Build history of the part. All positions in model axes, mm. A direction names the side the tool comes from. Round coordinates to 2 decimals unless told otherwise and drop trailing zeros. Write each loop counter-clockwise with the first axis right and the second up, starting at its lowest first coordinate (ties: lowest second). Pieces come first, ordered by that corner, then holes. Notation, with made-up numbers: (-20, 10.25) -> (2, 10.25) arc R19 cw to (2, 33.25) -> close; hole circle Ø1 at (53, -35). An arc over 180 degrees is marked (long way). Answer in a Markdown table with one row per item.
```python
from build123d import *

# Parameters (mm, degrees)
SKETCH1_R             = 3.81
BOSS_EXTRUDE1_DEPTH   = 127
F_2_64_TAPPED_HOLE1_D = 1.778
F_2_64_TAPPED_HOLE2_D = 1.778
LPATTERN1_COUNT       = 2
LPATTERN1_PITCH       = 25.4
LPATTERN2_COUNT       = 2
LPATTERN2_PITCH       = 25.4
SKETCH22_R            = 3.81
SKETCH22_R_2          = 2.38125
CUT_EXTRUDE1_DEPTH    = 12.7


with BuildPart() as part:
    # Sketch1 → Boss-Extrude1 (new body)
    with BuildSketch(Plane(origin=(0, 0, 0), x_dir=(1, 0, 0), z_dir=(0, 1, 0))):
        with Locations(Location((0, 0, 0), (0, 0, 270))):
            Circle(SKETCH1_R)
    extrude(amount=BOSS_EXTRUDE1_DEPTH)

    # #2-64 Tapped Hole1 (through all)
    with Locations(Plane(origin=(3.81, 0, 0), x_dir=(0, 0, -1), z_dir=(1, 0, 0))):
        with Locations((0, 76.2)):
            f_2_64_tapped_hole1 = Hole(F_2_64_TAPPED_HOLE1_D / 2)

    # #2-64 Tapped Hole2 (through all)
    with Locations(Plane(origin=(0, 0, 3.81), x_dir=(0, -1, 0), z_dir=(0, 0, 1))):
        with Locations((-88.9, 0)):
            f_2_64_tapped_hole2 = Hole(F_2_64_TAPPED_HOLE2_D / 2)

    # LPattern1: #2-64 Tapped Hole1 ×2
    with Locations(*[(0, i * LPATTERN1_PITCH, 0) for i in range(1, LPATTERN1_COUNT)]):
        add(f_2_64_tapped_hole1, mode=Mode.SUBTRACT)

    # LPattern2: #2-64 Tapped Hole2 ×2
    with Locations(*[(0, i * LPATTERN2_PITCH, 0) for i in range(1, LPATTERN2_COUNT)]):
        add(f_2_64_tapped_hole2, mode=Mode.SUBTRACT)

    # Sketch22 → Cut-Extrude1 (cut)
    with BuildSketch(Plane.XZ):
        with Locations(Location((0, 0, 0), (0, 0, 270))):
            Circle(SKETCH22_R)
        with Locations(Location((0, 0, 0), (0, 0, 270))):
            Circle(SKETCH22_R_2, mode=Mode.SUBTRACT)
    extrude(amount=-CUT_EXTRUDE1_DEPTH, mode=Mode.SUBTRACT)


solid = part.part
```
Q1. Which spindle directions (+Z, -Z, +X, -X, +Y, -Y) get a long thin tool onto all of the face, cutting with end or side? Do faces 1 (the flat face through (0, 0, 0)), 2 (the flat face through (-2, 12.7, 2)). Say none if no direction does.
A:
| item | result |
|---|---|
| face 1 | +Z, -Z, +X, -X, -Y |
| face 2 | -Y |
Q2. Drop flat-ended pins along their axis: P1, Ø2, axis at x = 0, y = 114.3, coming from the -Z side; P2, Ø2, axis at x = 2.5, y = 35, coming from the -Z side; P3, Ø2, axis at y = 83.5, z = 2, coming from the +X side. Give the stop position or say it passes through.
A:
| item | result |
|---|---|
| P1 | z = -3.81 |
| P2 | z = -3.5 |
| P3 | x = 3.68 |
Q3. Saw through at A-A on y = 55. Write the cut outline in (x, z).
A:
| item | result |
|---|---|
| outline | circle Ø7.62 at (0, 0) |
Q4. Wall check: line 1 (Y direction, x = 0, z = 2.25); line 2 (Y direction, x = -1.25, z = 0); line 3 (Z direction, x = 0, y = 101.5). Give the ranges that are in metal, low to high. Write a range as [from, to].
A:
| item | result |
|---|---|
| line 1 | [0, 88.01], [89.79, 113.41], [115.19, 127] |
| line 2 | [0, 75.31], [77.09, 100.71], [102.49, 127] |
| line 3 | [-3.81, -0.88], [0.88, 3.81] |
